```python
from build123d import *

# Parameters (mm, degrees)
F0_R     = 57.15
F1_DEPTH = 14.224
F2_R     = 7.112
F2_R_2   = 15.875
F3_DEPTH = 14.225
F5_DEPTH = 30.226


with BuildPart() as f1:
    # F0 (on Front) → F1 (new body)
    with BuildSketch(Plane.XZ):
        Circle(F0_R)
    extrude(amount=F1_DEPTH)

    # F2 (on face) → F3 (cut, through all)
    with BuildSketch(Plane.XZ.offset(14.224)):
        with Locations((0, -36.576)):
            Circle(F2_R)
        with Locations((31.675745, 18.288)):
            Circle(F2_R)
        with Locations((-31.675745, 18.288)):
            Circle(F2_R)
        Circle(F2_R_2)
    extrude(amount=-F3_DEPTH, mode=Mode.SUBTRACT)

    # F4 (on face) → F5 (join)
    with BuildSketch(Plane.XZ.offset(14.224)):
        with BuildLine():
            Line((20.723909, 31.970762), (36.762214, 35.059658))
            ThreePointArc((36.762214, 35.059658), (0, 50.8), (-36.762214, 35.059658))
            Line((-36.762214, 35.059658), (-20.723909, 31.970762))
            ThreePointArc((-20.723909, 31.970762), (0, 38.1), (20.723909, 31.970762))
        make_face()
        with BuildLine():
            Line((-38.049446, 1.962051), (-48.743661, 14.307182))
            ThreePointArc((-48.743661, 14.307182), (-43.994091, -25.4), (-11.981447, -49.36684))
            Line((-11.981447, -49.36684), (-17.325537, -33.932813))
            ThreePointArc((-17.325537, -33.932813), (-32.995568, -19.05), (-38.049446, 1.962051))
        make_face()
        with BuildLine():
            ThreePointArc((38.049446, 1.962051), (32.995568, -19.05), (17.325537, -33.932812))
            Line((17.325537, -33.932812), (11.981447, -49.36684))
            ThreePointArc((11.981447, -49.36684), (43.994091, -25.4), (48.743661, 14.307182))
            Line((48.743661, 14.307182), (38.049446, 1.962051))
        make_face()
    extrude(amount=F5_DEPTH)


solid = f1.part
```
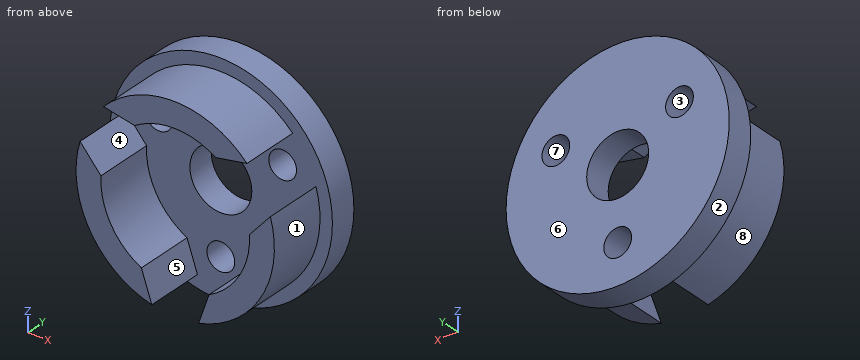
Input: part model. Units: mm. Frame: model coordinates. Face numbers are marked on the shaded views. A direction names the side the tool comes from. Give positions to 0.01 mm unless a question says otherwise; leave off trailing zeros. Order: outer loops, then holes, each group sorted by start corner. A loop starts at its lowest first (then second) coordinate and runs counter-clockwise, first axis right, second up. Notation, with made-up numbers: (-6.5, 23.5) -> (36.5, 23.5) arc R19 ccw to (36.5, 31.5) -> close; hole circle Ø10 at (-17, -15.5). An arc over 180 degrees is marked (long way). Write each question's results on one line, items separated by ' | '. Start each with the question number.
Item 1: Set-up query: the marked faces 4, 5, 6, 7 and 8. Return all of +Z, -Z, +X, -X, +Y, -Y with unobstructed straight access to the full face (end or side cutting, diameter ignored); none if empty.
Item 2: Cut plane B-B on x = 33. Return the cut outline in (y, z).
Item 3: Contact query for flat-ended pins moving along their axis: P1, Ø10, axis at x = -12.5, z = 16.5, coming from the -Y side; P2, Ø5, axis at x = 31.5, y = -23, coming from the -Z side; P3, Ø10, axis at y = -14, z = -16, coming from the -X side. Output: stop coordinate, or through.
Item 4: Cut plane A-A on z = 0. Return the cut outline in (x, y) (3 decimals), then the cut area to 3 significant figures.
Item 5: Mould query, pull axis X, two halves, no side actions, for the marked faces 1, 2 and 3. Classes: pulls with the +X half, pulls with the -X half, needs draft (parallel to the pull), parting line crosses it, or undercut.
Item 6: Cut plane D-D on x = 0. Return the cut outline in (y, z) (3 decimals), then the cut area to 3 significant figures.
Item 7: Cut plane C-C on y = -35.5. Return the cut outline in (x, z).
Item 8: Line query: line 1 (Y direction, x = -32.5, z = 0); line 2 (Z direction, x = 1.5, y = -13.5); line 3 (X direction, y = -25, z = 4). Output: solid intervals per line, ascending.
Established:
1) face 4: +Z, -Y | face 5: -Y | face 6: +Z, -Z, +X, -X, +Y | face 7: +Y, -Y | face 8: -X, -Y
2) outline: (-44.45, -38.62) -> (-14.22, -38.62) -> (-14.22, -46.66) -> (0, -46.66) -> (0, 11.3) -> (-14.22, 11.3) -> (-14.22, -19.04) -> (-44.45, -19.04) -> close; (-44.45, 34.34) -> (-14.22, 34.34) -> (-14.22, 25.28) -> (0, 25.28) -> (0, 46.66) -> (-14.22, 46.66) -> (-14.22, 38.62) -> (-44.45, 38.62) -> close
3) P1: y = -14.22 | P2: z = -41.71 | P3: x = -56.08
4) outline: (-57.15, -14.224) -> (-50.8, -14.224) -> (-50.8, -44.45) -> (-38.1, -44.45) -> (-38.1, -14.224) -> (-15.875, -14.224) -> (-15.875, 0) -> (-57.15, 0) -> close; (15.875, -14.224) -> (38.1, -14.224) -> (38.1, -44.45) -> (50.8, -44.45) -> (50.8, -14.224) -> (57.15, -14.224) -> (57.15, 0) -> (15.875, 0) -> close | area: 1,940 mm^2
5) face 1: pulls with the +X half | face 2: parting line crosses it | face 3: undercut
6) outline: (-44.45, 38.1) -> (-14.224, 38.1) -> (-14.224, 15.875) -> (0, 15.875) -> (0, 57.15) -> (-14.224, 57.15) -> (-14.224, 50.8) -> (-44.45, 50.8) -> close; (-14.224, -57.15) -> (0, -57.15) -> (0, -43.688) -> (-14.224, -43.688) -> close; (-14.224, -29.464) -> (0, -29.464) -> (0, -15.875) -> (-14.224, -15.875) -> close | area: 1,360 mm^2
7) outline: (-48.74, 14.31) arc R50.8 ccw to (-11.98, -49.37) -> (-17.33, -33.93) arc R38.1 cw to (-38.05, 1.96) -> close; (-36.76, 35.06) -> (-20.72, 31.97) arc R38.1 cw to (20.72, 31.97) -> (36.76, 35.06) arc R50.8 ccw to start; (11.98, -49.37) arc R50.8 ccw to (48.74, 14.31) -> (38.05, 1.96) arc R38.1 cw to (17.33, -33.93) -> close
8) line 1: -14.22 to 0 | line 2: -57.13 to -43.53, -29.62 to -15.8, 15.8 to 57.13 | line 3: -50.64 to -39.81, 39.81 to 50.64
